from build123d import *
from OCP.BRepFilletAPI import BRepFilletAPI_MakeChamfer

# Parameters (mm, degrees)
EXTRUDE_1_DEPTH     = 3
SKETCH_2_R          = 5.6
SKETCH_2_R_2        = 1.35
CUT_EXTRUDE_1_DEPTH = 95.288122264
CUT_EXTRUDE_2_DEPTH = 1.6
SKETCH_4_R          = 2.1
SKETCH_4_R_2        = 1.35
SKETCH_4_R_3        = 2
SKETCH_4_R_4        = 1.25
EXTRUDE_2_DEPTH     = 2
CHAMFER_1_SIZE      = 0.5
CHAMFER_1_SIZE2     = 0.288675135
FILLET_2_R          = 0.5


with BuildPart() as part:
    # 草圖1 → 填料-伸長1 (new body)
    with BuildSketch(Plane.XY):
        with BuildLine():
            Line((35.5, 33), (35.5, 29))
            ThreePointArc((35.5, 29), (36.085786438, 27.585786438), (37.5, 27))
            Line((37.5, 27), (85.5, 27))
            ThreePointArc((85.5, 27), (86.914213562, 26.414213562), (87.5, 25))
            Line((87.5, 25), (87.5, -25))
            ThreePointArc((87.5, -25), (86.914213562, -26.414213562), (85.5, -27))
            Line((85.5, -27), (37.5, -27))
            ThreePointArc((37.5, -27), (36.085786438, -27.585786438), (35.5, -29))
            Line((35.5, -29), (35.5, -33))
            ThreePointArc((35.5, -33), (34.914213562, -34.414213562), (33.5, -35))
            Line((33.5, -35), (-33.5, -35))
            ThreePointArc((-33.5, -35), (-34.914213562, -34.414213562), (-35.5, -33))
            Line((-35.5, -33), (-35.5, -29))
            ThreePointArc((-35.5, -29), (-36.085786438, -27.585786438), (-37.5, -27))
            Line((-37.5, -27), (-85.5, -27))
            ThreePointArc((-85.5, -27), (-86.914213562, -26.414213562), (-87.5, -25))
            Line((-87.5, -25), (-87.5, 25))
            ThreePointArc((-87.5, 25), (-86.914213562, 26.414213562), (-85.5, 27))
            Line((-85.5, 27), (-37.5, 27))
            ThreePointArc((-37.5, 27), (-36.085786438, 27.585786438), (-35.5, 29))
            Line((-35.5, 29), (-35.5, 33))
            ThreePointArc((-35.5, 33), (-34.914213562, 34.414213562), (-33.5, 35))
            Line((-33.5, 35), (33.5, 35))
            ThreePointArc((33.5, 35), (34.914213562, 34.414213562), (35.5, 33))
        make_face()
    extrude(amount=EXTRUDE_1_DEPTH)

    # 草圖2 → 除料-伸長1 (cut, through all)
    with BuildSketch(Plane.XY.offset(3)):
        Circle(SKETCH_2_R)
        with Locations((27, 6.25)):
            Circle(SKETCH_2_R_2)
        with Locations((6, 6.25)):
            Circle(SKETCH_2_R_2)
        with Locations((6, -6.25)):
            Circle(SKETCH_2_R_2)
        with Locations((27, -6.25)):
            Circle(SKETCH_2_R_2)
        with BuildLine():
            Line((43.45, -22.5), (43.45, 22.5))
            ThreePointArc((43.45, 22.5), (45, 24.05), (46.55, 22.5))
            Line((46.55, 22.5), (46.55, -22.5))
            ThreePointArc((46.55, -22.5), (45, -24.05), (43.45, -22.5))
        make_face()
        with BuildLine():
            Line((-46.55, -22.5), (-46.55, 22.5))
            ThreePointArc((-46.55, 22.5), (-45, 24.05), (-43.45, 22.5))
            Line((-43.45, 22.5), (-43.45, -22.5))
            ThreePointArc((-43.45, -22.5), (-45, -24.05), (-46.55, -22.5))
        make_face()
        with BuildLine():
            Line((21.5, -31.7), (8.5, -31.7))
            ThreePointArc((8.5, -31.7), (6.8, -30), (8.5, -28.3))
            Line((8.5, -28.3), (21.5, -28.3))
            ThreePointArc((21.5, -28.3), (23.2, -30), (21.5, -31.7))
        make_face()
        with BuildLine():
            Line((-21.5, -31.7), (-8.5, -31.7))
            ThreePointArc((-8.5, -31.7), (-6.8, -30), (-8.5, -28.3))
            Line((-8.5, -28.3), (-21.5, -28.3))
            ThreePointArc((-21.5, -28.3), (-23.2, -30), (-21.5, -31.7))
        make_face()
        with BuildLine():
            Line((21.5, 31.7), (8.5, 31.7))
            ThreePointArc((8.5, 31.7), (6.8, 30), (8.5, 28.3))
            Line((8.5, 28.3), (21.5, 28.3))
            ThreePointArc((21.5, 28.3), (23.2, 30), (21.5, 31.7))
        make_face()
        with BuildLine():
            Line((-21.5, 31.7), (-8.5, 31.7))
            ThreePointArc((-8.5, 31.7), (-6.8, 30), (-8.5, 28.3))
            Line((-8.5, 28.3), (-21.5, 28.3))
            ThreePointArc((-21.5, 28.3), (-23.2, 30), (-21.5, 31.7))
        make_face()
        with BuildLine():
            Line((21.5, 24.2), (8.5, 24.2))
            ThreePointArc((8.5, 24.2), (6.8, 22.5), (8.5, 20.8))
            Line((8.5, 20.8), (21.5, 20.8))
            ThreePointArc((21.5, 20.8), (23.2, 22.5), (21.5, 24.2))
        make_face()
        with BuildLine():
            Line((-21.5, 24.2), (-8.5, 24.2))
            ThreePointArc((-8.5, 24.2), (-6.8, 22.5), (-8.5, 20.8))
            Line((-8.5, 20.8), (-21.5, 20.8))
            ThreePointArc((-21.5, 20.8), (-23.2, 22.5), (-21.5, 24.2))
        make_face()
        with BuildLine():
            Line((-21.5, -24.2), (-8.5, -24.2))
            ThreePointArc((-8.5, -24.2), (-6.8, -22.5), (-8.5, -20.8))
            Line((-8.5, -20.8), (-21.5, -20.8))
            ThreePointArc((-21.5, -20.8), (-23.2, -22.5), (-21.5, -24.2))
        make_face()
        with BuildLine():
            Line((21.5, -24.2), (8.5, -24.2))
            ThreePointArc((8.5, -24.2), (6.8, -22.5), (8.5, -20.8))
            Line((8.5, -20.8), (21.5, -20.8))
            ThreePointArc((21.5, -20.8), (23.2, -22.5), (21.5, -24.2))
        make_face()
        with BuildLine():
            Line((-82.5, -17.5), (-82.5, -9.5))
            ThreePointArc((-82.5, -9.5), (-81, -8), (-79.5, -9.5))
            Line((-79.5, -9.5), (-79.5, -17.5))
            ThreePointArc((-79.5, -17.5), (-81, -19), (-82.5, -17.5))
        make_face()
        with BuildLine():
            Line((-82.5, 17.5), (-82.5, 9.5))
            ThreePointArc((-82.5, 9.5), (-81, 8), (-79.5, 9.5))
            Line((-79.5, 9.5), (-79.5, 17.5))
            ThreePointArc((-79.5, 17.5), (-81, 19), (-82.5, 17.5))
        make_face()
        with BuildLine():
            Line((79.5, -17.5), (79.5, -9.5))
            ThreePointArc((79.5, -9.5), (81, -8), (82.5, -9.5))
            Line((82.5, -9.5), (82.5, -17.5))
            ThreePointArc((82.5, -17.5), (81, -19), (79.5, -17.5))
        make_face()
        with BuildLine():
            Line((79.5, 17.5), (79.5, 9.5))
            ThreePointArc((79.5, 9.5), (81, 8), (82.5, 9.5))
            Line((82.5, 9.5), (82.5, 17.5))
            ThreePointArc((82.5, 17.5), (81, 19), (79.5, 17.5))
        make_face()
    extrude(amount=-CUT_EXTRUDE_1_DEPTH, mode=Mode.SUBTRACT)

    # 草圖3 → 除料-伸長2 (cut)
    with BuildSketch(Plane.XY.offset(3)):
        Polygon((29.482606158, -6.25), (28.241303079, -4.1), (25.758696921, -4.1), (24.517393842, -6.25), (25.758696921, -8.4), (28.241303079, -8.4), align=None)
        Polygon((8.482606158, -6.25), (7.241303079, -4.1), (4.758696921, -4.1), (3.517393842, -6.25), (4.758696921, -8.4), (7.241303079, -8.4), align=None)
        Polygon((29.482606158, 6.25), (28.241303079, 8.4), (25.758696921, 8.4), (24.517393842, 6.25), (25.758696921, 4.1), (28.241303079, 4.1), align=None)
        Polygon((8.482606158, 6.25), (7.241303079, 8.4), (4.758696921, 8.4), (3.517393842, 6.25), (4.758696921, 4.1), (7.241303079, 4.1), align=None)
    extrude(amount=-CUT_EXTRUDE_2_DEPTH, mode=Mode.SUBTRACT)

    # 草圖4 → 填料-伸長2 (add)
    # profile 1 of 4: a face of its own
    with BuildSketch(Plane(origin=(0, 0, 0), x_dir=(-1, 0, 0), z_dir=(0, 0, -1))):
        with Locations(Location((-27, 6.25, 0), (0, 0, 180))):
            Circle(SKETCH_4_R)
        with Locations(Location((-27, 6.25, 0), (0, 0, 180))):
            Circle(SKETCH_4_R_2, mode=Mode.SUBTRACT)
    # profile 2 of 4: a face of its own
    with BuildSketch(Plane(origin=(0, 0, 0), x_dir=(-1, 0, 0), z_dir=(0, 0, -1))):
        with Locations(Location((-27, -6.25, 0), (0, 0, 180))):
            Circle(SKETCH_4_R_3)
        with Locations((-27, -6.25)):
            Circle(SKETCH_4_R_4, mode=Mode.SUBTRACT)
    # profile 3 of 4: a face of its own
    with BuildSketch(Plane(origin=(0, 0, 0), x_dir=(-1, 0, 0), z_dir=(0, 0, -1))):
        with Locations(Location((-6, 6.25, 0), (0, 0, 180))):
            Circle(SKETCH_4_R_3)
        with Locations((-6, 6.25)):
            Circle(SKETCH_4_R_4, mode=Mode.SUBTRACT)
    # profile 4 of 4: a face of its own
    with BuildSketch(Plane(origin=(0, 0, 0), x_dir=(-1, 0, 0), z_dir=(0, 0, -1))):
        with Locations(Location((-6, -6.25, 0), (0, 0, 180))):
            Circle(SKETCH_4_R_3)
        with Locations((-6, -6.25)):
            Circle(SKETCH_4_R_4, mode=Mode.SUBTRACT)
    extrude(amount=EXTRUDE_2_DEPTH)

    # 導角1: one chamfer whose edges measure the first distance from different faces: ONE call of the kernel's chamfer builder (chamfer() names one face for all edges)
    chamfer_1_edges_1 = [part.edges().sort_by_distance(p)[0] for p in [
        (25.65, 6.25, -2),
    ]]
    chamfer_1_side_1 = [part.faces().sort_by_distance(p)[0] for p in [
        (24.95939697, 6.25, -2),
    ]]
    chamfer_1_edges_2 = [part.edges().sort_by_distance(p)[0] for p in [
        (28.25, -6.25, -2),
    ]]
    chamfer_1_side_2 = [part.faces().sort_by_distance(p)[0] for p in [
        (25.056568542, -6.25, -2),
    ]]
    chamfer_1_edges_3 = [part.edges().sort_by_distance(p)[0] for p in [
        (7.25, 6.25, -2),
    ]]
    chamfer_1_side_3 = [part.faces().sort_by_distance(p)[0] for p in [
        (4.056568542, 6.25, -2),
    ]]
    chamfer_1_edges_4 = [part.edges().sort_by_distance(p)[0] for p in [
        (7.25, -6.25, -2),
    ]]
    chamfer_1_side_4 = [part.faces().sort_by_distance(p)[0] for p in [
        (4.056568542, -6.25, -2),
    ]]
    chamfer_1 = BRepFilletAPI_MakeChamfer(part.part.solid().wrapped)
    for e in chamfer_1_edges_1:
        chamfer_1.Add(CHAMFER_1_SIZE, CHAMFER_1_SIZE2, e.wrapped, chamfer_1_side_1[0].wrapped)  # the first distance lies on this face
    for e in chamfer_1_edges_2:
        chamfer_1.Add(CHAMFER_1_SIZE, CHAMFER_1_SIZE2, e.wrapped, chamfer_1_side_2[0].wrapped)  # the first distance lies on this face
    for e in chamfer_1_edges_3:
        chamfer_1.Add(CHAMFER_1_SIZE, CHAMFER_1_SIZE2, e.wrapped, chamfer_1_side_3[0].wrapped)  # the first distance lies on this face
    for e in chamfer_1_edges_4:
        chamfer_1.Add(CHAMFER_1_SIZE, CHAMFER_1_SIZE2, e.wrapped, chamfer_1_side_4[0].wrapped)  # the first distance lies on this face
    add(Compound.cast(chamfer_1.Shape()), mode=Mode.REPLACE)

    # 圓角2
    fillet_2_edges = [part.edges().sort_by_distance(p)[0] for p in [
        (24.9, 6.25, 0),
        (25, -6.25, 0),
        (4, 6.25, 0),
        (4, -6.25, 0),
    ]]
    fillet(fillet_2_edges, radius=FILLET_2_R)


solid = part.part
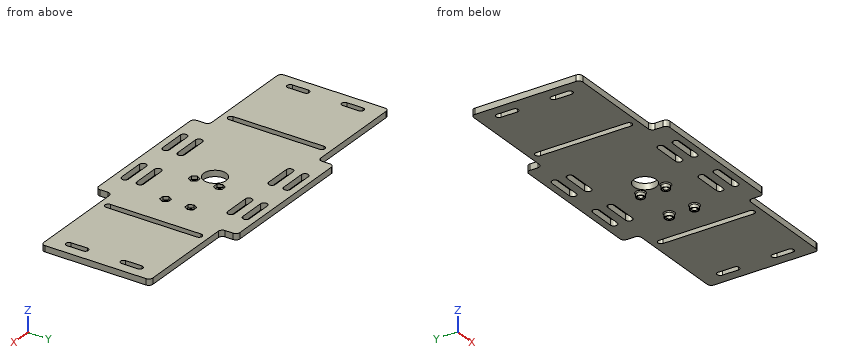
Work out the finished part from the listing and answer in its coordinate system (mm). Give positions to 0.01 mm unless a question says otherwise; leave off trailing zeros. Loops run counter-clockwise (first coordinate to the right, second up) from the corner with the lowest first, then second, coordinate; pieces in that order, holes last. Notation, with made-up numbers: (-2, -39.75) -> (54, -39.75) arc R14 ccw to (54, -28.75) -> close; hole circle Ø8 at (-28.5, -21). An arc over 180 degrees is marked (long way). Use a Markdown table: item, result. Add a question column.
1. Section B-B on x = 0 is taken. Determine the outline of the cut face in (y, z).
2. Find the intervals of material crossed by probe 1 along Y at (x, z) = (6, 0.55); probe 2 along X at (y, z) = (-9.5, 2.6); probe 3 along Y at (x, z) = (-11.5, 0.75), in increasing order.
3. Section A-A on y = 0 is taken. Determine the outline of the cut face in (x, z).
4. Section C-C on x = 66 is taken. Determine the outline of the cut face in (y, z), and give its area (3 significant figures).
5. Flat-ended cylindrical pins translate along their axes: pin 1 Ø1.3 at (x, y) = (6.5, -7) entering from +Z; pin 2 Ø4.5 at (x, y) = (26.5, -5.5) entering from +Z; pin 3 Ø6 at (x, y) = (-47, 6) entering from -Z; pin 4 Ø2 at (x, y) = (6, 6.25) entering from -Z. Find the tip coordinate at first contact, or state that the pin passes through.
Results below:
| question | item | result |
|---|---|---|
| 1 | outline | (-35, 0) -> (-5.6, 0) -> (-5.6, 3) -> (-35, 3) -> close; (5.6, 0) -> (35, 0) -> (35, 3) -> (5.6, 3) -> close |
| 2 | probe 1 | y = -35 to -7.6, -4.9 to 4.9, 7.6 to 35 |
| 2 | probe 2 | x = -87.5 to -82.5, -79.5 to -46.55, -43.45 to 43.45, 46.55 to 79.5, 82.5 to 87.5 |
| 2 | probe 3 | y = -35 to -31.7, -28.3 to -24.2, -20.8 to 20.8, 24.2 to 28.3, 31.7 to 35 |
| 3 | outline | (-87.5, 0) -> (-46.55, 0) -> (-46.55, 3) -> (-87.5, 3) -> close; (-43.45, 0) -> (-5.6, 0) -> (-5.6, 3) -> (-43.45, 3) -> close; (5.6, 0) -> (43.45, 0) -> (43.45, 3) -> (5.6, 3) -> close; (46.55, 0) -> (87.5, 0) -> (87.5, 3) -> (46.55, 3) -> close |
| 4 | outline | (-27, 0) -> (27, 0) -> (27, 3) -> (-27, 3) -> close |
| 4 | area | 162 mm^2 |
| 5 | pin 1 | stops at z = 1.4 |
| 5 | pin 2 | stops at z = 3 |
| 5 | pin 3 | stops at z = 0 |
| 5 | pin 4 | passes through |
